from build123d import *

# Parameters (mm, degrees)
SKETCH1_W           = 139.7
SKETCH1_H           = 200.02
BOSS_EXTRUDE1_DEPTH = 3.18
SKETCH2_R           = 1.5
SKETCH2_W           = 3.18
SKETCH2_H           = 90.135
CUT_EXTRUDE1_DEPTH  = 4.18
SKETCH5_W           = 88.895716174
SKETCH5_H           = 168.56277979
BOSS_EXTRUDE2_DEPTH = 3.18
SKETCH6_W           = 20
SKETCH6_H           = 200.02
BOSS_EXTRUDE3_DEPTH = 3.18
SKETCH7_W           = 56.795
SKETCH7_H           = 3.18
CUT_EXTRUDE4_DEPTH  = 4.18
SKETCH8_W           = 133.34
SKETCH8_H           = 1.59
CUT_EXTRUDE5_DEPTH  = 4.18
SKETCH9_R           = 1.6
CUT_EXTRUDE6_DEPTH  = 4.18
SKETCH10_W          = 24.565797096
SKETCH10_H          = 10.537213664
CUT_EXTRUDE7_DEPTH  = 3.18
SKETCH11_R          = 1.59
SKETCH11_R_2        = 1.71788268
CUT_EXTRUDE8_DEPTH  = 35
SKETCH12_W          = 3.18
SKETCH12_H          = 3.18
CUT_EXTRUDE9_DEPTH  = 80.725


with BuildPart() as part:
    # Sketch1 → Boss-Extrude1 (new body)
    with BuildSketch(Plane.XY):
        Rectangle(SKETCH1_W, SKETCH1_H)
    extrude(amount=BOSS_EXTRUDE1_DEPTH)

    # Sketch2 → Cut-Extrude1 (cut, through all)
    with BuildSketch(Plane.XY.offset(3.18)):
        with Locations((-67.85, 0)):
            Circle(SKETCH2_R)
        with Locations((67.85, 0)):
            Circle(SKETCH2_R)
        Polygon((-10, 100.01), (10, 100.01), (10, 96.83), (1.5, 96.83), (1.5, 92.83), (3.5, 92.83), (3.5, 89.83), (1.5, 89.83), (1.5, 86.83), (-1.5, 86.83), (-1.5, 89.83), (-3.5, 89.83), (-3.5, 92.83), (-1.5, 92.83), (-1.5, 96.83), (-10, 96.83), align=None)
        Polygon((-10, -100.01), (-10, -96.83), (-1.5, -96.83), (-1.5, -92.83), (-3.5, -92.83), (-3.5, -89.83), (-1.5, -89.83), (-1.5, -86.83), (1.5, -86.83), (1.5, -89.83), (3.5, -89.83), (3.5, -92.83), (1.5, -92.83), (1.5, -96.83), (10, -96.83), (10, -100.01), align=None)
        with Locations((-68.26, 54.9425)):
            Rectangle(SKETCH2_W, SKETCH2_H)
        with Locations((-68.26, -54.9425)):
            Rectangle(SKETCH2_W, SKETCH2_H)
        with Locations((68.26, -54.9425)):
            Rectangle(SKETCH2_W, SKETCH2_H)
        with Locations((68.26, 54.9425)):
            Rectangle(SKETCH2_W, SKETCH2_H)
    extrude(amount=-CUT_EXTRUDE1_DEPTH, mode=Mode.SUBTRACT)

    # Sketch5 → Boss-Extrude2 (add)
    with BuildSketch(Plane.XY.offset(3.18)):
        Rectangle(SKETCH5_W, SKETCH5_H)
    extrude(amount=-BOSS_EXTRUDE2_DEPTH)

    # Sketch6 → Boss-Extrude3 (add)
    with BuildSketch(Plane.XY.offset(3.18)):
        Rectangle(SKETCH6_W, SKETCH6_H)
    extrude(amount=-BOSS_EXTRUDE3_DEPTH)

    # Sketch7 → Cut-Extrude4 (cut, through all)
    with BuildSketch(Plane.XY.offset(3.18)):
        with Locations((-38.2725, -98.42)):
            Rectangle(SKETCH7_W, SKETCH7_H)
        with Locations((38.2725, -98.42)):
            Rectangle(SKETCH7_W, SKETCH7_H)
    extrude(amount=-CUT_EXTRUDE4_DEPTH, mode=Mode.SUBTRACT)

    # Sketch8 → Cut-Extrude5 (cut, through all)
    with BuildSketch(Plane.XY.offset(3.18)):
        with Locations((0, 99.215)):
            Rectangle(SKETCH8_W, SKETCH8_H)
    extrude(amount=-CUT_EXTRUDE5_DEPTH, mode=Mode.SUBTRACT)

    # Sketch9 → Cut-Extrude6 (cut, through all)
    with BuildSketch(Plane.XY.offset(3.18)):
        with Locations((-52.981261278, 49.292856132)):
            Circle(SKETCH9_R)
        with Locations((-4.68387739, 47.615742656)):
            Circle(SKETCH9_R)
        with Locations((-20.064964891, -3.1597647)):
            Circle(SKETCH9_R)
        with Locations((-47.964929331, -3.115219713)):
            Circle(SKETCH9_R)
    extrude(amount=-CUT_EXTRUDE6_DEPTH, mode=Mode.SUBTRACT)

    # Sketch10 → Cut-Extrude7 (cut)
    with BuildSketch(Plane.XY.offset(3.18)):
        with Locations((-3.359789788, -56.149532718)):
            Rectangle(SKETCH10_W, SKETCH10_H)
    extrude(amount=-CUT_EXTRUDE7_DEPTH, mode=Mode.SUBTRACT)

    # Sketch11 → Cut-Extrude8 (cut)
    with BuildSketch(Plane.XY.offset(3.18)):
        with Locations((17.523878239, 81.797398404)):
            Circle(SKETCH11_R)
        with Locations((-14.883091948, 81.797398404)):
            Circle(SKETCH11_R_2)
    extrude(amount=-CUT_EXTRUDE8_DEPTH, mode=Mode.SUBTRACT)

    # Sketch12 → Cut-Extrude9 (cut, through all)
    with BuildSketch(Plane.ZY.offset(9.875)):
        with Locations((1.59, -98.42)):
            Rectangle(SKETCH12_W, SKETCH12_H)
    extrude(amount=-CUT_EXTRUDE9_DEPTH, mode=Mode.SUBTRACT)


solid = part.part
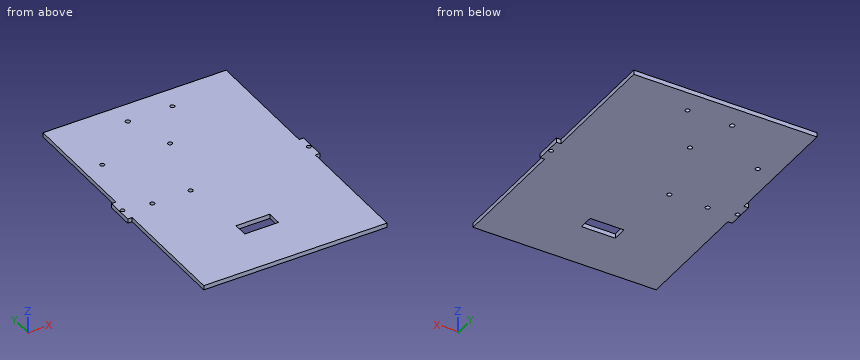
Here's how the part is built. I have some questions about the finished solid (model axes, mm). Give positions to 0.01 mm unless a question says otherwise; leave off trailing zeros. Order: outer loops, then holes, each group sorted by start corner. A loop starts at its lowest first (then second) coordinate and runs counter-clockwise, first axis right, second up. Notation, with made-up numbers: (17.25, -39) -> (71.25, -39) arc R17 cw to (71.25, -31) -> close; hole circle Ø3 at (39, 2.25). An arc over 180 degrees is marked (long way). One line per item, written item: value. Start each with the question number.
1. Imagine slicing it at B-B, the plane z = 2. Count the separate pieces of the cut face and the enclosed holes in it, plus the area to 3 significant figures.
2. Will these pins go through, and if not, where does the flat tip stop? pin 1 Ø1 at (x, z) = (-69, 1.5) entering from -Y (3 decimals); pin 2 Ø1.5 at (y, z) = (-66.5, 1.5) entering from -X.
3. Imagine slicing it at A-A, the plane x = 2. List the corners of the cut face in (y, z) for me, plus the area to 3 significant figures.
4. I need wall thicknesses on probe 1 along X at (y, z) = (83, 1.35); probe 2 along X at (y, z) = (-55, 0.25); probe 3 along Y at (x, z) = (-20, 2.65). Which ranges of each line are inside material? Lowest first, please. Write a range as from..to.
5. Imagine slicing it at C-C, the plane y = 59.5. List the corners of the cut face in (x, z) for me.
Values follow:
1. separate pieces: 1
1. enclosed holes: 9
1. area: 25,800 mm2
2. pin 1: stops at y = -9.875
2. pin 2: stops at x = -66.67
3. outline: (-96.83, 0) -> (-61.42, 0) -> (-61.42, 3.18) -> (-96.83, 3.18) -> close; (-50.88, 0) -> (98.42, 0) -> (98.42, 3.18) -> (-50.88, 3.18) -> close
3. area: 587 mm2
4. probe 1: x = -66.67..-16.11, -13.66..16.48, 18.56..66.67
4. probe 2: x = -66.67..-15.64, 8.92..66.67
4. probe 3: y = -96.83..-4.76, -1.56..98.42
5. outline: (-66.67, 0) -> (66.67, 0) -> (66.67, 3.18) -> (-66.67, 3.18) -> close
